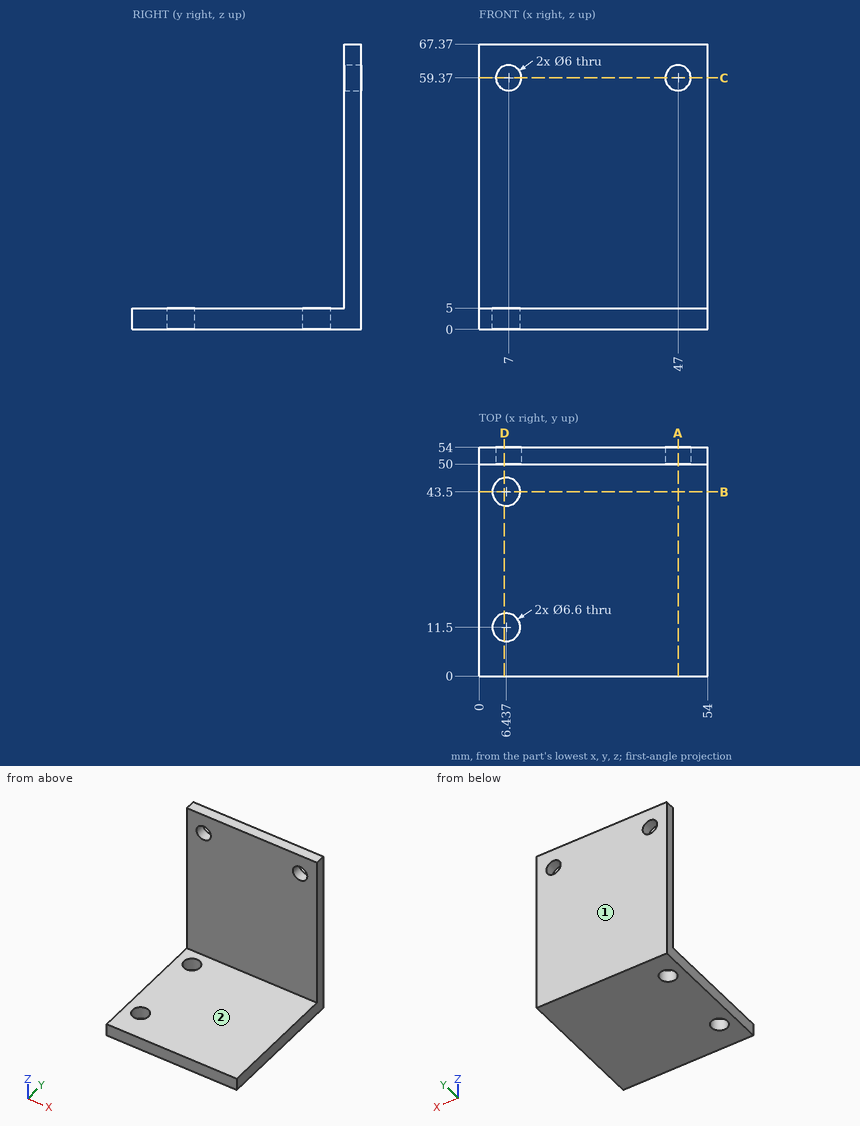
Geometry: see drawing. Coordinates: mm, zero at the bounding-box minimum. A direction names the side the tool comes from. Round coordinates to 2 decimals unless told otherwise and drop trailing zeros. Write each loop counter-clockwise with the first axis right and the second up, starting at its lowest first coordinate (ties: lowest second). Pieces come first, ordered by that corner, then holes.
1) Cut plane A-A (x = 47). Return the cut outline in (y, z).
2) Cut plane C-C (z = 59.37). Return the cut outline in (x, y).
3) Cut plane D-D (x = 6). Return the cut outline in (y, z).
4) Contact query for flat-ended pins moving along their axis: P1, Ø5, axis at x = 47, z = 59.37, coming from the +Y side; P2, Ø8.5, axis at x = 6.44, y = 11.5, coming from the -Z side; P3, Ø9.5, axis at x = 7, z = 59.37, coming from the -Y side; P4, Ø4, axis at x = 16.5, y = 45, coming from the +Z side. Output: stop coordinate, or through.
5) Cut plane B-B (y = 43.5). Return the cut outline in (x, z).
6) Reachability of the marked faces 1 and 2 from +Z, -Z, +X, -X, +Y, -Y: full face, straight path, thin tool, end or side. Return the list, or none.
7) Ray query, L1, parallel to X at y = 53, z = 59.37; L2, parallel to Z at x = 33, y = 31.5; L3, parallel to Y at x = 38, z = 46.5. Return the intervals inside material, ascending.
Geometry says:
1. outline: (0, 0) - (54, 0) - (54, 56.37) - (50, 56.37) - (50, 5) - (0, 5) - close; (50, 62.37) - (54, 62.37) - (54, 67.37) - (50, 67.37) - close
2. outline: (0, 50) - (4, 50) - (4, 54) - (0, 54) - close; (10, 50) - (44, 50) - (44, 54) - (10, 54) - close; (50, 50) - (54, 50) - (54, 54) - (50, 54) - close
3. outline: (0, 0) - (8.23, 0) - (8.23, 5) - (0, 5) - close; (14.77, 0) - (40.23, 0) - (40.23, 5) - (14.77, 5) - close; (46.77, 0) - (54, 0) - (54, 56.54) - (50, 56.54) - (50, 5) - (46.77, 5) - close; (50, 62.2) - (54, 62.2) - (54, 67.37) - (50, 67.37) - close
4. P1: passes through
4. P2: stops at z = 0
4. P3: stops at y = 50
4. P4: stops at z = 5
5. outline: (0, 0) - (3.14, 0) - (3.14, 5) - (0, 5) - close; (9.74, 0) - (54, 0) - (54, 5) - (9.74, 5) - close
6. face 1: +Z, -Z, +X, -X, +Y
6. face 2: +Z, +X, -X, -Y
7. L1: x = 0 to 4, 10 to 44, 50 to 54
7. L2: z = 0 to 5
7. L3: y = 50 to 54
